Verification items for the finished model (mm, model axes). Coordinates: 2 decimals unless noted, no trailing zeros. Write each loop counter-clockwise with the first axis right and the second up, starting at its lowest first coordinate (ties: lowest second). Pieces come first, ordered by that corner, then holes. Notation, with made-up numbers: (34, 54.25) -> (61, 54.25) arc R23 cw to (61, 66.25) -> close; hole circle Ø4 at (52, 21.5). An arc over 180 degrees is marked (long way). Answer in a Markdown table with one row per item.
Autodesk Inventor part; units mm, degrees
ref_plane "YZ Plane" through (0, 0, 0) normal (1, 0, 0) x (0, 1, 0)
ref_plane "XZ Plane" through (0, 0, 0) normal (0, 1, 0) x (-1, 0, 0)
ref_plane "XY Plane" through (0, 0, 0) normal (0, 0, 1) x (1, 0, 0)
sketch "スケッチ1" plane through (0, 0, 0) normal (0, 1, 0) x (-1, 0, 0)
  circle A0 centre (0, 0) radius 4.6188 construction
  line L0 (4.6188, 0) -> (2.3094, 4)
  line L1 (2.3094, 4) -> (-2.3094, 4)
  line L2 (-2.3094, 4) -> (-4.6188, 0)
  line L3 (-4.6188, 0) -> (-2.3094, -4)
  line L4 (-2.3094, -4) -> (2.3094, -4)
  line L5 (2.3094, -4) -> (4.6188, 0)
  dimension "d0" = 8
extrude "押し出し1" add sketch "スケッチ1" along normal blind 4
sketch "スケッチ2" plane through (0, 4, 0) normal (0, 1, 0) x (1, 0, 0)
  point P0 (0, 0)
  point P1 (0, 0)
hole "穴1" at (0, 4, 0) direction (0, -1, 0) diameter 4.134 end through all
sketch "スケッチ3" plane through (0, 0, 0) normal (1, 0, 0) x (0, 1, 0)
  arc A0 (3.1544, -5) -> (4, -4) centre (-1.7446, 0) ccw
  line L0 (0, -4) -> (4, -4) construction
  line L1 (4, -5) -> (3.1544, -5)
  line L2 (4, 2.067) -> (4, -2.067) construction
  line L3 (4, -4) -> (4, -5)
  line L4 (-4.0084, 0) -> (4.4272, 0)
  point P0 (0, 0)
  point P1 (4, 0)
  dimension "d10" = 4
  dimension "d11" = 7
  dimension "d12" = 1
revolve "回転1" cut sketch "スケッチ3" angle 360 about axis through (0, -10, 0) along (0, 1, 0)
properties part number "M3-HexaNut-type2"
1. Release check for a two-part mould opening along X. For faces 1 (the face through (1.26, 1.97, -1.64)), 2 (the face through (-1, 0, 2)), 3 (the face through (3.448, 1.972, 2.028)) record: released by +X, released by -X, zero draft, split by the parting line, or undercut.
Findings below:
| item | result |
|---|---|
| face 1 | undercut |
| face 2 | zero draft |
| face 3 | released by +X |
2. Material ranges on probe 1 along Z at (x, y) = (0, 2.05); probe 2 along X at (y, z) = (1.25, 1.5); probe 3 along X at (y, z) = (0.8, 0.25), recorded low to high. Write a range as from..to.
Findings below:
| item | result |
|---|---|
| probe 1 | z = -4..-2.07, 2.07..4 |
| probe 2 | x = -3.75..-1.42, 1.42..3.75 |
| probe 3 | x = -4.47..-2.05, 2.05..4.47 |
3. Go/stop test with flat-tipped pins: pin 1 (1.5 mm diameter, centred on y = 1.5, z = -2, fed in from -X); pin 2 (4 mm diameter, centred on x = 2, z = 1, fed in from -Y). Record where each tip stops, or that it passes through.
Findings below:
| item | result |
|---|---|
| pin 1 | stops at x = -3.9 |
| pin 2 | stops at y = 0 |
4. Sectioned sample at A-A, the plane y = 1. Record the cut outline in (x, z).
Findings below:
| item | result |
|---|---|
| outline | (-4.62, 0) -> (-2.31, -4) -> (2.31, -4) -> (4.62, 0) -> (2.31, 4) -> (-2.31, 4) -> close; hole circle Ø4.13 at (0, 0) |
